Read the model definition and answer for the solid it produces. Units are mm, in the model's axes. A direction names the side the tool comes from. Round coordinates to 2 decimals unless told otherwise and drop trailing zeros. Order: outer loops, then holes, each group sorted by start corner. A loop starts at its lowest first (then second) coordinate and runs counter-clockwise, first axis right, second up. Notation, with made-up numbers: M 49,-16 L 76,-16 A22 cw 76,14 Z; hole C -35,12 d9. An arc over 180 degrees is marked long. Use one line per item in the form item = value. Start each with the question number.
from build123d import *

# Parameters (mm, degrees)
F1_DEPTH = 30
F3_D     = 6.8
F3_DEPTH = 3.201
F5_D     = 5
F5_DEPTH = 6.2
F5_TIP   = 1.5021515476


with BuildPart() as f1:
    # F0 (on Front) → F1 (new body)
    with BuildSketch(Plane.XZ):
        Polygon((80, 0), (0, 0), (0, 30), (69.2820323028, 70), (67.6820323028, 72.7712812921), (-3.2, 31.8475208614), (-3.2, -3.2), (80, -3.2), align=None)
    extrude(amount=-F1_DEPTH)

    # F3 (through all, one way)
    with BuildSketch(Plane.XY):
        with Locations((35, 15), (65, 15)):
            Circle(F3_D / 2)
    extrude(amount=-F3_DEPTH, mode=Mode.SUBTRACT)

    # F5
    with Locations(Plane(origin=(-14.5903810568, 0, 25.2712812921), x_dir=(0.8660254038, 0, 0.5), z_dir=(-0.5, 0, 0.8660254038))):
        with Locations((75, 15), (45, 15)):
            Hole(F5_D / 2, depth=F5_DEPTH)
            with Locations((0, 0, -(F5_DEPTH + F5_TIP / 2))):  # 118° drill point
                Cone(0, F5_D / 2, F5_TIP, mode=Mode.SUBTRACT)


solid = f1.part
Item 1: For a pull along Y with two mould halves and no side action, classify faces 4 (the cylindrical face through (52.89, 13.48, 62.36)), 5 (the flat face through (22.8, 0, 43.4)), 6 (the flat face through (22.8, 30, 43.4)) as pulls with the +Y half, pulls with the -Y half, needs draft (parallel to the pull), parting line crosses it, or undercut.
Item 2: Section C-C (x = 35) is taken. Write down the section's boundary in (y, z), and give its area (3 significant figures).
Item 3: Find the intervals of material crossed by L1, parallel to Y at x = 65, z = -2; L2, parallel to Z at x = 53.5, y = 16.5; L3, parallel to Z at x = 16.5, y = 26.75, in increasing order. Write a range as [from, to].
Item 4: Section D-D (y = 16) is taken. Write down the section's boundary in (x, z), and give its area (3 significant figures).
Item 5: Section B-B (x = 10) is taken. Write down the section's boundary in (y, z), and give its area (3 significant figures).
Item 6: Given P1, Ø4, axis at y = 8.5, z = 42.5, coming from the +X side; P2, Ø3, axis at x = 61, y = 19, coming from the +Z side; P3, Ø4, axis at x = 35, y = 15, coming from the +Z side, each flat-ended and moving along its own axis, determine where each tip first touches the part or whether it passes through.
Item 7: Section A-A (y = 27) is taken. Write down the section's boundary in (x, z), and give its area (3 significant figures).
Item 8: A tool of negligible diameter and unlimited length cuts with its end or side. For faces 1 (the flat face through (38, 11, -3.2)), 2 (the flat face through (41, 15, 0)), 3 (the cylindrical face through (68.14, 13.7, -1.58)), from which of +Z, -Z, +X, -X, +Y, -Y can it reach the whole face along a straight path? Write none if from no direction.
The answers:
q1.face_4 = undercut
q1.face_5 = pulls with the -Y half
q1.face_6 = pulls with the +Y half
q2.outline = M 0,-3.2 L 11.6,-3.2 L 11.6,0 L 0,0 Z; M 0,50.21 L 30,50.21 L 30,53.9 L 0,53.9 Z; M 18.4,-3.2 L 30,-3.2 L 30,0 L 18.4,0 Z
q2.area = 185 mm²
q3.L1 = [0, 11.6], [18.4, 30]
q3.L2 = [-3.2, 0], [61.34, 64.58]
q3.L3 = [-3.2, 0], [39.53, 43.22]
q4.outline = M -3.2,-3.2 L 31.75,-3.2 L 31.75,0 L 0,0 L 0,30 L 24,43.85 L 22.4,46.63 L -3.2,31.85 Z; M 26.37,48.92 L 27.97,46.15 L 49.98,58.85 L 48.38,61.63 Z; M 38.25,-3.2 L 61.75,-3.2 L 61.75,0 L 38.25,0 Z; M 52.35,63.92 L 53.95,61.15 L 69.28,70 L 67.68,72.77 Z; M 68.25,-3.2 L 80,-3.2 L 80,0 L 68.25,0 Z
q4.area = 553 mm²
q5.outline = M 0,-3.2 L 30,-3.2 L 30,0 L 0,0 Z; M 0,35.77 L 30,35.77 L 30,39.47 L 0,39.47 Z
q5.area = 207 mm²
q6.P1 = 25.11
q6.P2 = 69.78
q6.P3 = 55.06
q7.outline = M -3.2,-3.2 L 80,-3.2 L 80,0 L 0,0 L 0,30 L 69.28,70 L 67.68,72.77 L -3.2,31.85 Z
q7.area = 624 mm²
q8.face_1 = -Z, +X, -X, +Y, -Y
q8.face_2 = +X, +Y, -Y
q8.face_3 = -Z
